Verification items for the finished model (mm, model axes). A direction names the side the tool comes from. Coordinates: 2 decimals unless noted, no trailing zeros. Order: outer loops, then holes, each group sorted by start corner. A loop starts at its lowest first (then second) coordinate and runs counter-clockwise, first axis right, second up.
Q1. Cross-section at C-C, the plane y = -9.5. Record the boundary of the cut face in (x, z) (3 decimals), and give its area (3 significant figures).
Q2. Set-up check for faces 4 (the flat face through (0, -2, -30)), 5 (the flat face through (0, -3, 25.8)), 6 (the flat face through (0, -1, -27.8)): record each of +Z, -Z, +X, -X, +Y, -Y from which the full face is reachable in a straight line by a thin tool's end or side.
Q3. Cross-section at B-B, the plane z = -15. Record the boundary of the cut face in (x, y) (3 decimals).
Q4. Depth check by flat-ended pin: P1, Ø1.6, axis at x = -9, z = -26.5, coming from the -Y side; P2, Ø3, axis at x = 2, z = -29.5, coming from the -Y side; P3, Ø2, axis at x = -17.75, z = -32.8, coming from the +Y side. Enter the tip coordinate at first touch or a pass-through.
Q5. Thickness scan on line 1 (X direction, y = -1.55, z = -32.8) (3 decimals); line 2 (Z direction, x = 0, y = -1) (3 decimals); line 3 (Z direction, x = 10, y = -3.5). Record the ranges inside material, lowest first.
Q6. Draft check along Z on faces 1 (the flat face through (0, -11, -37.8)), 2 (the flat face through (0, -11, 28.838)), 3 (the flat face through (0, -4, -27)). Enter one of: pulls with the +Z half, pulls with the -Z half, needs draft (parallel to the pull), parting line crosses it, or undercut.
Autodesk Inventor part; units mm, degrees
ref_plane "YZ Plane" through (0, 0, 0) normal (1, 0, 0) x (0, 1, 0)
ref_plane "XY Plane" through (0, 0, 0) normal (0, 0, 1) x (1, 0, 0)
sketch "Sketch1" plane through (0, 0, 0) normal (0, 1, 0) x (-1, 0, 0)
  line L0 (24.775, -25.7234) -> (-24.775, -25.7234)
  line L1 (-24.775, -25.7234) -> (-24.775, 25.7234)
  line L2 (-24.775, 25.7234) -> (24.775, 25.7234)
  line L3 (24.775, 25.7234) -> (24.775, -25.7234)
  line L4 (24.775, -25.7234) -> (-24.775, 25.7234) construction
  line L5 (-24.775, -25.7234) -> (24.775, 25.7234) construction
  line L6 (26.775, -27.8) -> (-26.775, -27.8)
  line L7 (-26.775, -27.8) -> (-26.775, 27.8)
  line L8 (-26.775, 27.8) -> (26.775, 27.8)
  line L9 (26.775, 27.8) -> (26.775, -27.8)
  line L10 (26.775, -27.8) -> (-26.775, 27.8) construction
  line L11 (-26.775, -27.8) -> (26.775, 27.8) construction
  line L12 (-26.775, -17.5745) -> (-24.775, -17.5745)
  line L13 (27.775, -28.8383) -> (-27.775, -28.8383)
  line L14 (-27.775, -28.8383) -> (-27.775, 28.8383)
  line L15 (-27.775, 28.8383) -> (27.775, 28.8383)
  line L16 (27.775, 28.8383) -> (27.775, -28.8383)
  line L17 (27.775, -28.8383) -> (-27.775, 28.8383) construction
  line L18 (-27.775, -28.8383) -> (27.775, 28.8383) construction
  line L19 (-27.775, -9.8151) -> (-26.775, -9.8151)
  line L20 (-7.9068, 27.8) -> (-7.9068, 28.8383)
  line L21 (27.775, -27.8) -> (27.775, -37.8)
  line L22 (27.775, -37.8) -> (-27.775, -37.8)
  line L23 (-27.775, -37.8) -> (-27.775, -27.8)
  line L24 (27.775, -37.8) -> (27.775, -32.8)
  line L25 (27.775, -32.8) -> (-27.775, -32.8)
  line L26 (27.775, -32.8) -> (15.7648, -32.8)
  line L27 (27.775, -32.8) -> (17.75, -32.8)
  circle A0 centre (17.75, -32.8) radius 1.825
  line L28 (-27.775, -32.8) -> (-17.75, -32.8)
  circle A1 centre (-17.75, -32.8) radius 1.825
  circle A2 centre (0, -32.8) radius 1.825
  point P0 (0, 0)
  point P1 (22.7625, -32.8)
  point P2 (21.7699, -32.8)
  point P3 (-22.7625, -32.8)
  point P4 (-27.775, -28.8383)
  dimension "d0" = 53.55
  dimension "d1" = 55.6
  dimension "d2" = 2
  dimension "d3" = 1
  dimension "d4" = 10
  dimension "d6" = 55.55
  dimension "d8" = 10.025
  dimension "d9" = 3.65
  dimension "d11" = 10.025
  dimension "d12" = 3.65
  dimension "d13" = 3.65
extrude "Extrusion1" add sketch "Sketch1" against normal blind 25 contours L7 L6 L9 L8 L20 L15 L16 L13 L14 L19 | L19 L14 L15 L20 L8 L7 | L13 L21 L25 A0 A2 A1 L23 | L25 A1 A2 A0 L21 L22 L23
sketch "Sketch2" plane through (0, -25, 0) normal (0, -1, 0) x (1, 0, 0)
  line L0 (-26.775, -27.8) -> (-26.775, -36.8)
  line L1 (26.775, -27.8) -> (-26.775, -27.8)
  line L2 (-26.775, -36.8) -> (26.775, -36.8)
  line L3 (26.775, -36.8) -> (26.775, -27.8)
  line L4 (26.775, -27.8) -> (-26.775, -27.8)
  line L5 (-26.775, -27.8) -> (-26.775, -36.8)
  point P0 (0, 0)
  dimension "d16" = 9
extrude "Extrusion2" cut sketch "Sketch2" against normal blind 23
ref_plane "Work Plane1" through (0, -2, 0) normal (0, 1, 0) x (-1, 0, 0)
sketch "Sketch3" plane through (0, -2, 0) normal (0, 1, 0) x (-1, 0, 0)
  line L0 (26.775, -27.8) -> (-26.775, -27.8)
  line L1 (-26.775, -27.8) -> (-26.775, 27.8)
  line L2 (26.775, -27.8) -> (-26.775, -27.8)
  line L3 (-26.775, -27.8) -> (-26.775, 27.8)
  line L4 (-26.775, 27.8) -> (26.775, 27.8)
  line L5 (26.775, 27.8) -> (26.775, -27.8)
  line L6 (24.75, 25.8) -> (-24.75, 25.8)
  line L7 (-24.75, 25.8) -> (-24.75, -25.8)
  line L8 (-24.75, -25.8) -> (24.75, -25.8)
  line L9 (24.75, -25.8) -> (24.75, 25.8)
  line L10 (24.75, 25.8) -> (-24.75, -25.8) construction
  line L11 (-24.75, 25.8) -> (24.75, -25.8) construction
  point P0 (0, 0)
  dimension "d20" = 49.5
  dimension "d21" = 51.6
extrude "Extrusion3" add sketch "Sketch3" against normal blind 2
sketch "Sketch4" plane through (0, -4, 0) normal (0, -1, 0) x (1, 0, 0)
  line L0 (24.75, -25.8) -> (24.75, 25.8)
  line L1 (-26.775, -27.8) -> (26.775, -27.8)
  line L2 (24.75, -25.8) -> (26.775, -25.8)
  line L3 (26.775, -25.8) -> (26.775, -27.8)
  line L4 (26.775, -27.8) -> (24.75, -27.8)
  line L5 (24.75, -27.8) -> (24.75, -25.8)
  line L6 (24.75, 25.8) -> (-24.75, 25.8)
  line L7 (-26.775, 27.8) -> (26.775, 27.8)
  line L8 (24.75, 25.8) -> (26.775, 25.8)
  line L9 (26.775, 25.8) -> (26.775, 27.8)
  line L10 (26.775, 27.8) -> (24.75, 27.8)
  line L11 (24.75, 27.8) -> (24.75, 25.8)
  line L12 (-24.75, 25.8) -> (-26.775, 25.8)
  line L13 (-26.775, 25.8) -> (-26.775, 27.8)
  line L14 (-26.775, 27.8) -> (-24.75, 27.8)
  line L15 (-24.75, 27.8) -> (-24.75, 25.8)
  line L16 (-24.75, -25.8) -> (-24.75, 25.8)
  line L17 (-24.75, -25.8) -> (-26.775, -25.8)
  line L18 (-26.775, -25.8) -> (-26.775, -27.8)
  line L19 (-26.775, -27.8) -> (-24.75, -27.8)
  line L20 (-24.75, -27.8) -> (-24.75, -25.8)
  point P0 (0, 0)
extrude "Extrusion4" add sketch "Sketch4" along normal blind 21 contours L2 L3 L1 L5 | L11 L7 L9 L8 | L12 L13 L7 L15 | L1 L18 L17 L20
sketch "Sketch5" plane through (27.775, 0, -37.8) normal (0, 0, -1) x (-1, 0, 0)
  line L0 (52.525, -25) -> (3.025, -25)
  line L1 (0, 0) -> (55.55, 0)
  line L2 (27.775, -18) -> (32.275, -18)
  line L3 (27.775, -18) -> (23.275, -18)
  line L4 (23.275, -18) -> (23.275, -22.5)
  line L5 (32.275, -18) -> (32.275, -22.5)
  line L6 (23.275, -22.5) -> (32.275, -22.5)
  point P0 (27.775, 0)
  point P1 (27.775, 0)
  dimension "d29" = 4.5
  dimension "d30" = 4.5
  dimension "d34" = 4.5
  dimension "d35" = 4.5
sketch "Sketch6" plane through (0, -25, 0) normal (0, -1, 0) x (1, 0, 0)
  line L0 (-27.775, -37.8) -> (27.775, -37.8)
  line L1 (27.775, -37.8) -> (27.775, 28.8383)
  line L2 (-27.775, -37.8) -> (27.775, -37.8)
  line L3 (27.775, -37.8) -> (27.775, 28.8383)
  line L4 (27.775, 28.8383) -> (-27.775, 28.8383)
  line L5 (-27.775, 28.8383) -> (-27.775, -37.8)
  point P0 (0, 0)
extrude "Extrusion5" cut sketch "Sketch6" against normal blind 2
extrude "Extrusion6" cut sketch "Sketch5" against normal blind 2
properties part number "Mainbody2"
Check values:
1. outline: (-27.775, -37.8) - (27.775, -37.8) - (27.775, 28.838) - (-27.775, 28.838) - close; hole (-26.775, -36.8) - (26.775, -36.8) - (26.775, -27.8) - (24.75, -27.8) - (24.75, -25.8) - (26.775, -25.8) - (26.775, 25.8) - (24.75, 25.8) - (24.75, 27.8) - (-24.75, 27.8) - (-24.75, 25.8) - (-26.775, 25.8) - (-26.775, -25.8) - (-24.75, -25.8) - (-24.75, -27.8) - (-26.775, -27.8) - close
1. area: 259 mm2
2. face 4: -Y
2. face 5: +Y, -Y
2. face 6: +Y
3. outline: (-27.775, -23) - (-26.775, -23) - (-26.775, -4) - (-24.75, -4) - (-24.75, -2) - (-26.775, -2) - (-26.775, 0) - (-27.775, 0) - close; (24.75, -4) - (26.775, -4) - (26.775, -23) - (27.775, -23) - (27.775, 0) - (26.775, 0) - (26.775, -2) - (24.75, -2) - close
4. P1: stops at y = -4
4. P2: stops at y = -2
4. P3: passes through
5. line 1: x = -27.775 to -19.575, -15.925 to -1.825, 1.825 to 15.925, 19.575 to 27.775
5. line 2: z = -37.8 to -34.625, -30.975 to -27.8, 27.8 to 28.838
5. line 3: z = -37.8 to -36.8, -27.8 to -25.8, 25.8 to 28.84
6. face 1: pulls with the -Z half
6. face 2: pulls with the +Z half
6. face 3: undercut
